Read the model definition and answer for the solid it produces. Units are mm, in the model's axes. A direction names the side the tool comes from. Coordinates: 2 decimals unless noted, no trailing zeros. Loops run counter-clockwise (first coordinate to the right, second up) from the corner with the lowest first, then second, coordinate; pieces in that order, holes last. Notation, with made-up numbers: (-24, 27) - (21, 27) arc R24 ccw to (21, 64) - close; hole circle Ø5 at (56, 80). An arc over 180 degrees is marked (long way). Use CSV: the item, a comma, the result in double quotes.
Autodesk Inventor part; units mm, degrees
ref_plane "Work Plane1" through (29, 0, 0) normal (0, -1, 0) x (1, 0, 0)
ref_plane "YZ Plane" through (0, 0, 0) normal (1, 0, 0) x (0, 1, 0)
ref_plane "XZ Plane" through (0, 0, 0) normal (0, 1, 0) x (-1, 0, 0)
sketch "Sketch1" plane through (0, 0, 0) normal (0, 0, 1) x (1, 0, 0)
  line L0 (-0.0762, 0) -> (6.35, 0)
  line L1 (6.35, 0) -> (6.35, 1.7526)
  line L2 (6.35, 1.7526) -> (1.5902, 1.7526)
  line L3 (1.5902, 1.7526) -> (0.0001, 1.7526)
  line L4 (0.0001, 1.7526) -> (0, 1.7526)
  line L5 (0, 1.7526) -> (0, 3.3274)
  line L6 (0, 3.3274) -> (-1.8542, 3.3274)
  line L7 (-1.8542, 3.3274) -> (-1.8542, 1.1438)
  line L8 (-1.8542, 1.1438) -> (-0.7366, 1.1438)
  line L9 (-0.7366, 1.1438) -> (-0.0762, 0)
  line L10 (-3.495, 0) -> (7.9908, 0)
  line L11 (0, -0.6655) -> (0, 3.9929)
  line L12 (1.5902, 1.7526) -> (0, 1.7526) construction
  dimension "d1" = 4.7598
  dimension "d2" = 1.5901
  dimension "d3" = 1.8542
  dimension "d4" = 1.1176
  dimension "d5" = 60
  dimension "d6" = 3.5052
  dimension "d7" = 3.5052
  dimension "d8" = 2.2877
  dimension "d9" = 6.6548
  dimension "d26" = 6.35
revolve "Body" add sketch "Sketch1" angle 360 about axis through (-0.0762, 0, 0) along (1, 0, 0)
sketch "Sketch2" plane through (-1.8542, 0, 0) normal (-1, 0, 0) x (0, 0, 1)
  circle A0 centre (0, 0) radius 1.1438
  line L0 (0, -4.6584) -> (0, 4.6584)
  line L1 (-4.6584, 0) -> (4.6584, 0)
  line L2 (1.1438, 0) -> (0.5719, -0.9906)
  line L3 (0.5719, -0.9906) -> (-0.5719, -0.9906)
  line L4 (-0.5719, -0.9906) -> (-1.1438, 0)
  line L5 (-1.1438, 0) -> (-0.5719, 0.9906)
  line L6 (-0.5719, 0.9906) -> (0.5719, 0.9906)
  line L7 (0.5719, 0.9906) -> (1.1438, 0)
  point P0 (0, 0)
extrude "Slot" add sketch "Sketch2" against normal up to next contours L7 A0 | A0 L2 | L6 L0 A0 | A0 L0 L3 | L0 L6 A0 | A0 L3 L0 | L4 A0 | A0 L5
fillet "Fillet1" radius 1.6002 1 edges at (-1.8542, -3.3274, 0)
thread "Thread"
chamfer "Chamfer1" distance 0.4869 distance2 0.4869 1 edges at (6.35, -1.7526, 0) measured on face at (6.35, -0.5672, -0.1398)
ref_plane "Work Plane1" through (29, 0, 0) normal (0, -1, 0) x (1, 0, 0)
fillet "Fillet2" radius 0.1 1 edges at (0.0001, -1.7526, 0)
equation "\"d1\" = GEL"
equation "\"d3\" = KOH"
equation "\"d4\" = INTI"
equation "\"d6\" = GD"
equation "\"d7\" = BDM"
equation "\"d8\" = 1.1547 * SW"
equation "\"d9\" = KOD"
equation "\"d26\" = NLG"
equation "\"d30\" = R"
equation "\"d17\" = RR"
equation "\"d13\" = GEL"
equation "\"d15\" = -0.5 * SPD + 0.5 * GD"
equation "\"d16\" = GUL"
equation "\"GD\" = NND"
equation "\"NLG\" = 6.35"
equation "\"GEL\" = 4.75976"
equation "\"KOD\" = 6.6548"
equation "\"KOH\" = 1.8542"
equation "\"INTI\" = 1.1176"
equation "\"GAL\" = 1.59004"
equation "\"GUL\" = 0.48692"
equation "\"BDM\" = NND"
equation "\"SW\" = 1.9812"
equation "\"RR\" = 1.6002"
equation "\"SPD\" = 2.53136"
equation "\"R\" = 0.1"
equation "\"TOA\" = 30deg"
equation "\"GD1\" = SPD"
equation "\"THREADDIA\" = 3.5052"
equation "\"KOH1\" = 0.381"
equation "\"NND\" = 3.5052"
equation "\"E0\" = 2.28829"
properties part number "ANSI B18.3 - 6 - 32 x 1/4" material "Steel, Mild"
Q1. For a pull along Y with two mould halves and no side action, classify faces 3 (the face through (2.94, 1.67, -0.53)), 4 (the face through (0, 1, 2)), 5 (the face through (-1.26, -0.49, 0.86)) as +Y half, -Y half, draft (parallel to the pull), parting line (faces both ways), or undercut.
Reported:
face 3,"parting line"
face 4,"draft"
face 5,"undercut"
Q2. The part is cut by section C-C on x = -0.5. Determine the outline of the cut face in (y, z), and give its area (3 significant figures).
Reported:
outline,"circle Ø6.62 at (0, 0); hole circle Ø1.47 at (0, 0)"
area,"32.7 mm²"
Q3. Given P1, Ø2, axis at x = 3.5, z = 1.5, coming from the +Y side; P2, Ø1.3, axis at x = -1.5, z = 0, coming from the +Y side; P3, Ø1, axis at x = 0, z = 2, coming from the -Y side, each flat-ended and moving along its own axis, determine where each tip first touches the part or whether it passes through.
Reported:
P1,"stops at y = 1.68"
P2,"stops at y = 3.21"
P3,"stops at y = -2.97"
Q4. The part is cut by section A-A on x = -1.5. Determine the outline of the cut face in (y, z).
Reported:
outline,"circle Ø5.46 at (0, 0); hole (-0.99, -0.57) - (0, -1.14) - (0.99, -0.57) - (0.99, 0.57) - (0, 1.14) - (-0.99, 0.57) - close"
Q5. The part is cut by section B-B on x = 4. Determine the outline of the cut face in (y, z).
Reported:
outline,"circle Ø3.51 at (0, 0)"
Q6. A tool of negligible diameter and unlimited length cuts with its end or side. For faces 1 (the face through (-1, 0.991, 0)), 2 (the face through (-1.854, -1, 1)), from which of +Z, -Z, +X, -X, +Y, -Y can it reach the whole face along a straight path? Write none if from no direction.
Reported:
face 1,"-X"
face 2,"+Z, -Z, -X, +Y, -Y"
Q7. Find the intervals of material crossed by probe 1 along Z at (x, y) = (-0.5, -0.5); probe 2 along Y at (x, z) = (3.75, -0.5); probe 3 along Z at (x, y) = (-1, 2), in increasing order. Write a range as [from, to].
Reported:
probe 1,"z = [-3.27, -0.54], [0.54, 3.27]"
probe 2,"y = [-1.68, 1.68]"
probe 3,"z = [-2.42, 2.42]"
